Part model, mm, in its own coordinate system. A direction names the side the tool comes from. Round coordinates to 2 decimals unless told otherwise and drop trailing zeros. Order: outer loops, then holes, each group sorted by start corner. A loop starts at its lowest first (then second) coordinate and runs counter-clockwise, first axis right, second up. Notation, with made-up numbers: M 84.25,71.5 L 95.25,71.5 A30 cw 95.25,100.5 Z; hole C 41.25,-24 d2. An arc over 180 degrees is marked long. Write each question's results on one line, items separated by ' | '. Start each with the question number.
1. Band-saw the part on A-A, the plane z = 0.45. List the corners of the cut face in (x, y).
2. Drop flat-ended pins along their axis: pin 1 Ø0.8 at (y, z) = (1, -0.5) entering from +X; pin 2 Ø4.5 at (x, y) = (6, 0) entering from +Z; pin 3 Ø0.5 at (y, z) = (-1.5, -0.5) entering from -X; pin 4 Ø1.1 at (y, z) = (4.5, 3.5) entering from +X. Give the stop position or say it passes through.
3. Two-plate mould, pull along X, no slides. Class faces 1 (the face through (-3, -1.5, -0.4)), 2 (the face through (0, -5, 2)), 3 (the face through (-7.75, 0.08, 2.46)): +X half, -X half, draft (parallel to the pull), parting line (faces both ways), or undercut.
4. Which spindle directions (+Z, -Z, +X, -X, +Y, -Y) get a long thin tool onto all of the face, cutting with end or side? Do faces 4 (the face through (-3, 2.5, -0.4)), 5 (the face through (3, 0.5, -0.4)), 6 (the face through (3, 4.5, 2.5)). Say none if no direction does.
5. Band-saw the part on C-C, the plane x = -1.75. List the corners of the cut face in (y, z), then the cut area to 3 significant figures.
6. Band-saw the part on D-D, the plane x = 5. List the corners of the cut face in (y, z), then the cut area to 3 significant figures.
7. Probe L1, parallel to Y at x = 6, z = 3.2; L2, parallel to X at y = 1, z = 3.4; L3, parallel to X at y = 0.5, z = 2. List the from-to ranges inside material, lowest first. Write a range as [from, to].
8. Band-saw the part on B-B, the plane y = 0.25. List the corners of the cut face in (x, z).
```python
from build123d import *

# Parameters (mm, degrees)
SKETCH1_R           = 1.75
BOSS_EXTRUDE1_DEPTH = 5
SKETCH2_W           = 6
SKETCH2_H           = 1
BOSS_EXTRUDE2_DEPTH = 1
FILLET1_START       = -3
FILLET1_DEPTH       = 6
FILLET1_2_DEPTH     = 6


with BuildPart() as part:
    # Sketch1 → Boss-Extrude1 (new body)
    with BuildSketch(Plane.XY):
        with BuildLine():
            Line((-6, 5), (-3, 5))
            Line((-3, 5), (-3, 4))
            Line((-3, 4), (3, 4))
            Line((3, 4), (3, 5))
            Line((3, 5), (6, 5))
            ThreePointArc((6, 5), (8.828427125, 3.828427125), (10, 1))
            Line((10, 1), (10, -1))
            ThreePointArc((10, -1), (8.828427125, -3.828427125), (6, -5))
            Line((6, -5), (-6, -5))
            ThreePointArc((-6, -5), (-8.828427125, -3.828427125), (-10, -1))
            Line((-10, -1), (-10, 1))
            ThreePointArc((-10, 1), (-8.828427125, 3.828427125), (-6, 5))
        make_face()
        with Locations((6, 0)):
            Circle(SKETCH1_R, mode=Mode.SUBTRACT)
        with Locations((-6, 0)):
            Circle(SKETCH1_R, mode=Mode.SUBTRACT)
    extrude(amount=BOSS_EXTRUDE1_DEPTH)

    # Sketch2 → Boss-Extrude2 (add)
    with BuildSketch(Plane(origin=(0, 0, 0), x_dir=(-1, 0, 0), z_dir=(0, 0, -1))):
        with Locations((0, 2.5)):
            Rectangle(SKETCH2_W, SKETCH2_H)
        with Locations((0, 0.5)):
            Rectangle(SKETCH2_W, SKETCH2_H)
        with Locations((0, -1.5)):
            Rectangle(SKETCH2_W, SKETCH2_H)
        with Locations((0, -3.5)):
            Rectangle(SKETCH2_W, SKETCH2_H)
    extrude(amount=BOSS_EXTRUDE2_DEPTH)

    # Fillet1: read off the stored shape, not the designer's step
    # Fillet1 outline → Fillet1 (cut)
    with BuildSketch(Plane.YZ.offset(FILLET1_START)):
        with BuildLine():
            ThreePointArc((-3.5, -1), (-3.853553391, -0.853553391), (-4, -0.5))
            Line((-4, -0.5), (-4, -1))
            Line((-4, -1), (-3.5, -1))
        make_face()
        with BuildLine():
            ThreePointArc((-3, -0.5), (-3.146446609, -0.853553391), (-3.5, -1))
            Line((-3.5, -1), (-3, -1))
            Line((-3, -1), (-3, -0.5))
        make_face()
        with BuildLine():
            ThreePointArc((-1.5, -1), (-1.853553391, -0.853553391), (-2, -0.5))
            Line((-2, -0.5), (-2, -1))
            Line((-2, -1), (-1.5, -1))
        make_face()
        with BuildLine():
            ThreePointArc((-1, -0.5), (-1.146446609, -0.853553391), (-1.5, -1))
            Line((-1.5, -1), (-1, -1))
            Line((-1, -1), (-1, -0.5))
        make_face()
        with BuildLine():
            ThreePointArc((0.5, -1), (0.146446609, -0.853553391), (0, -0.5))
            Line((0, -0.5), (0, -1))
            Line((0, -1), (0.5, -1))
        make_face()
        with BuildLine():
            ThreePointArc((1, -0.5), (0.853553391, -0.853553391), (0.5, -1))
            Line((0.5, -1), (1, -1))
            Line((1, -1), (1, -0.5))
        make_face()
        with BuildLine():
            ThreePointArc((2.5, -1), (2.146446609, -0.853553391), (2, -0.5))
            Line((2, -0.5), (2, -1))
            Line((2, -1), (2.5, -1))
        make_face()
        with BuildLine():
            ThreePointArc((3, -0.5), (2.853553391, -0.853553391), (2.5, -1))
            Line((2.5, -1), (3, -1))
            Line((3, -1), (3, -0.5))
        make_face()
    extrude(amount=FILLET1_DEPTH, mode=Mode.SUBTRACT)

    # Fillet1 2 outline → Fillet1 2 (add)
    with BuildSketch(Plane.YZ.offset(FILLET1_START)):
        with BuildLine():
            Line((-4, 0), (-4.5, 0))
            ThreePointArc((-4.5, 0), (-4.146446609, -0.146446609), (-4, -0.5))
            Line((-4, -0.5), (-4, 0))
        make_face()
        with BuildLine():
            Line((2, 0), (1.5, 0))
            ThreePointArc((1.5, 0), (1.853553391, -0.146446609), (2, -0.5))
            Line((2, -0.5), (2, 0))
        make_face()
        with BuildLine():
            Line((0, 0), (-0.5, 0))
            ThreePointArc((-0.5, 0), (-0.146446609, -0.146446609), (0, -0.5))
            Line((0, -0.5), (0, 0))
        make_face()
        with BuildLine():
            Line((-2, 0), (-2.5, 0))
            ThreePointArc((-2.5, 0), (-2.146446609, -0.146446609), (-2, -0.5))
            Line((-2, -0.5), (-2, 0))
        make_face()
        with BuildLine():
            Line((-2.5, 0), (-3, 0))
            Line((-3, 0), (-3, -0.5))
            ThreePointArc((-3, -0.5), (-2.853553391, -0.146446609), (-2.5, 0))
        make_face()
        with BuildLine():
            Line((-0.5, 0), (-1, 0))
            Line((-1, 0), (-1, -0.5))
            ThreePointArc((-1, -0.5), (-0.853553391, -0.146446609), (-0.5, 0))
        make_face()
        with BuildLine():
            Line((1.5, 0), (1, 0))
            Line((1, 0), (1, -0.5))
            ThreePointArc((1, -0.5), (1.146446609, -0.146446609), (1.5, 0))
        make_face()
        with BuildLine():
            Line((3.5, 0), (3, 0))
            Line((3, 0), (3, -0.5))
            ThreePointArc((3, -0.5), (3.146446609, -0.146446609), (3.5, 0))
        make_face()
    extrude(amount=FILLET1_2_DEPTH)


solid = part.part
```
Solution:
1) outline: M -10,-1 A4 ccw -6,-5 L 6,-5 A4 ccw 10,-1 L 10,1 A4 ccw 6,5 L 3,5 L 3,4 L -3,4 L -3,5 L -6,5 A4 ccw -10,1 Z; hole C -6,0 d3.5; hole C 6,0 d3.5
2) pin 1: x = 3 | pin 2: z = 5 | pin 3: x = -3 | pin 4: x = 8.7
3) face 1: -X half | face 2: draft | face 3: undercut
4) face 4: -Z, -X, +Y, -Y | face 5: -Z, +X, +Y, -Y | face 6: +Z, -Z, +Y
5) outline: M -5,0 L -4.5,0 A0.5 cw -4,-0.5 A0.5 ccw -3,-0.5 A0.5 cw -2,-0.5 A0.5 ccw -1,-0.5 A0.5 cw 0,-0.5 A0.5 ccw 1,-0.5 A0.5 cw 2,-0.5 A0.5 ccw 3,-0.5 A0.5 cw 3.5,0 L 4,0 L 4,5 L -5,5 Z | area: 49.0 mm^2
6) outline: M -5,0 L -1.44,0 L -1.44,5 L -5,5 Z; M 1.44,0 L 5,0 L 5,5 L 1.44,5 Z | area: 35.6 mm^2
7) L1: [-5, -1.75], [1.75, 5] | L2: [-10, -7.44], [-4.56, 4.56], [7.44, 10] | L3: [-10, -7.68], [-4.32, 4.32], [7.68, 10]
8) outline: M -10,0 L -7.73,0 L -7.73,5 L -10,5 Z; M -4.27,0 L -3,0 L -3,-0.93 L 3,-0.93 L 3,0 L 4.27,0 L 4.27,5 L -4.27,5 Z; M 7.73,0 L 10,0 L 10,5 L 7.73,5 Z
